For this review, use the dimensioned drawing (mm, ordinates from the lowest corner) and the shaded views. A direction names the side the tool comes from. Give positions to 0.01 mm unless a question says otherwise; leave off trailing zeros. Order: outer loops, then holes, each group sorted by start corner. A loop starts at its lowest first (then second) coordinate and runs counter-clockwise, first axis right, second up. Notation, with made-up numbers: M 53.5,61 L 60.5,61 A29 cw 60.5,91 Z; hole C 16,28 d7. An arc over 180 degrees is marked long. Use CSV: the item, a comma, the result in double quotes. Start each with the question number.
(1) Consider section C-C (y = 3.75). Write out the cut boundary in (x, z).
(2) Tool access review of the marked faces 1 and 2: name each direction out of +Z, -Z, +X, -X, +Y, -Y from which nothing blocks a thin tool from reaching the whole face with its end or side.
(3) Wall thickness on L1, parallel to Z at x = 32.5, y = 5.5; L2, parallel to X at y = 8.75, z = 32.5; L3, parallel to Y at x = 37, z = 54.5: over which ranges is each line inside the solid? List them lowest first. Write a range as from..to.
(4) Clearance check with flat-ended pins moving along their axes: P1, Ø3, axis at x = 32.5, z = 32.5, coming from the +Y side; P2, Ø2, axis at x = 30, y = 4, coming from the +Z side; P3, Ø5, axis at x = 27, y = 10.5, coming from the +Z side; P4, Ø8, axis at x = 25.5, y = 8, coming from the +Z side. State where each tip first meets the part, or that it passes through.
(5) Consider section B-B (x = 32.5). Write out the cut boundary in (y, z), and give its area (3 significant figures).
(6) Consider section A-A (z = 32.5). Write out the cut boundary in (x, y), and give its area (4 significant figures).
(7) Consider section D-D (x = 21.5). Write out the cut boundary in (y, z).
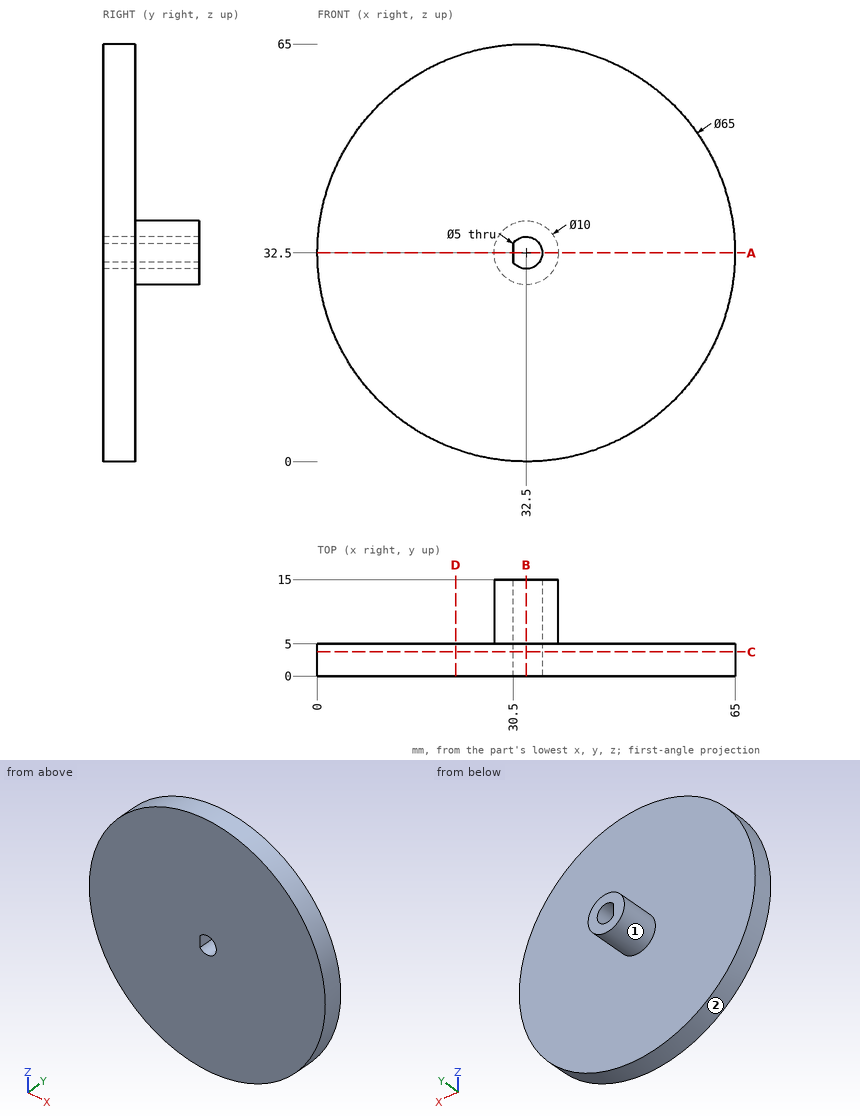
Check result:
1,outline,"C 32.5,32.5 d65; hole M 30.5,31 A2.5 ccw long 30.5,34 Z"
2,face 1,"+Y"
2,face 2,"+Y, -Y"
3,L1,"z = 27.5..30, 35..37.5"
3,L2,"x = 27.5..30.5, 35..37.5"
3,L3,"y = 0..5"
4,P1,"passes through"
4,P2,"stops at z = 64.97"
4,P3,"stops at z = 36.5"
4,P4,"stops at z = 64.71"
5,outline,"M 0,0 L 5,0 L 5,27.5 L 15,27.5 L 15,30 L 0,30 Z; M 0,35 L 15,35 L 15,37.5 L 5,37.5 L 5,65 L 0,65 Z"
5,area,"350 mm^2"
6,outline,"M 0,0 L 30.5,0 L 30.5,15 L 27.5,15 L 27.5,5 L 0,5 Z; M 35,0 L 65,0 L 65,5 L 37.5,5 L 37.5,15 L 35,15 Z"
6,area,"357.5 mm^2"
7,outline,"M 0,1.92 L 5,1.92 L 5,63.08 L 0,63.08 Z"
